Can you work these out from the drawing? Everything is in mm from the part's minimum corner. A direction names the side the tool comes from. Give positions to 0.01 mm unless a question says otherwise; leave off trailing zeros. Loops run counter-clockwise (first coordinate to the right, second up) from the corner with the lowest first, then second, coordinate; pieces in that order, holes last.
Q1. If we section it at C-C (y = 2.3): Please give me the cut outline in (x, z), plus the area to 3 significant figures.
Q2. For the marked faces 1, 2, 3 and 4, which set-ups out of +Z, -Z, +X, -X, +Y, -Y let a thin tool reach every point of the face, with its end or its side?
Q3. I need wall thicknesses on line 1 (Y direction, x = 1.3, z = 2.6); line 2 (Z direction, x = 4.9, y = 0.6); line 3 (Z direction, x = 1.15, y = 1.65). Which ranges of each line are inside material? Lowest first, please.
Q4. Will these pins go through, and if not, where does the flat tip stop? P1, Ø2, axis at x = 1.5, y = 5.5, coming from the +Z side; P2, Ø1.6, axis at y = 4.5, z = 2.5, coming from the -X side; P3, Ø3, axis at x = 1.5, y = 1.5, coming from the +Z side; P4, Ø1, axis at x = 3, z = 4.5, coming from the -Y side.
Q5. If we section it at D-D (z = 4.55): Please give me the cut outline in (x, y).
Q6. If we section it at A-A (x = 2.6): Please give me the cut outline in (y, z).
Q7. If we section it at B-B (z = 3.05): Please give me the cut outline in (x, y).
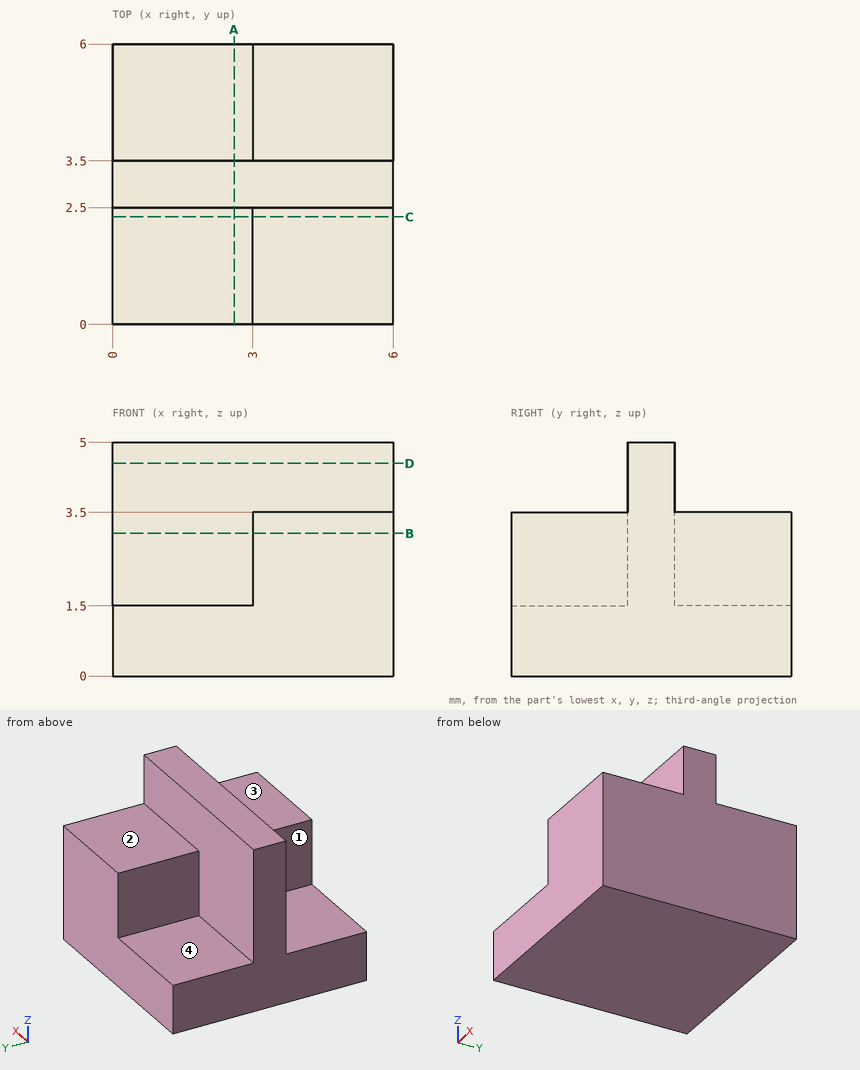
Check sheet entries:
1. outline: (0, 0) - (6, 0) - (6, 3.5) - (3, 3.5) - (3, 1.5) - (0, 1.5) - close
1. area: 15.0 mm2
2. face 1: +Z, -X, -Y
2. face 2: +Z, +X, -X, +Y
2. face 3: +Z, +X, -X, -Y
2. face 4: +Z, -X, +Y
3. line 1: y = 2.5 to 3.5
3. line 2: z = 0 to 3.5
3. line 3: z = 0 to 1.5
4. P1: stops at z = 1.5
4. P2: stops at x = 3
4. P3: stops at z = 5
4. P4: stops at y = 2.5
5. outline: (0, 2.5) - (6, 2.5) - (6, 3.5) - (0, 3.5) - close
6. outline: (0, 0) - (6, 0) - (6, 1.5) - (3.5, 1.5) - (3.5, 5) - (2.5, 5) - (2.5, 1.5) - (0, 1.5) - close
7. outline: (0, 2.5) - (3, 2.5) - (3, 0) - (6, 0) - (6, 6) - (3, 6) - (3, 3.5) - (0, 3.5) - close
